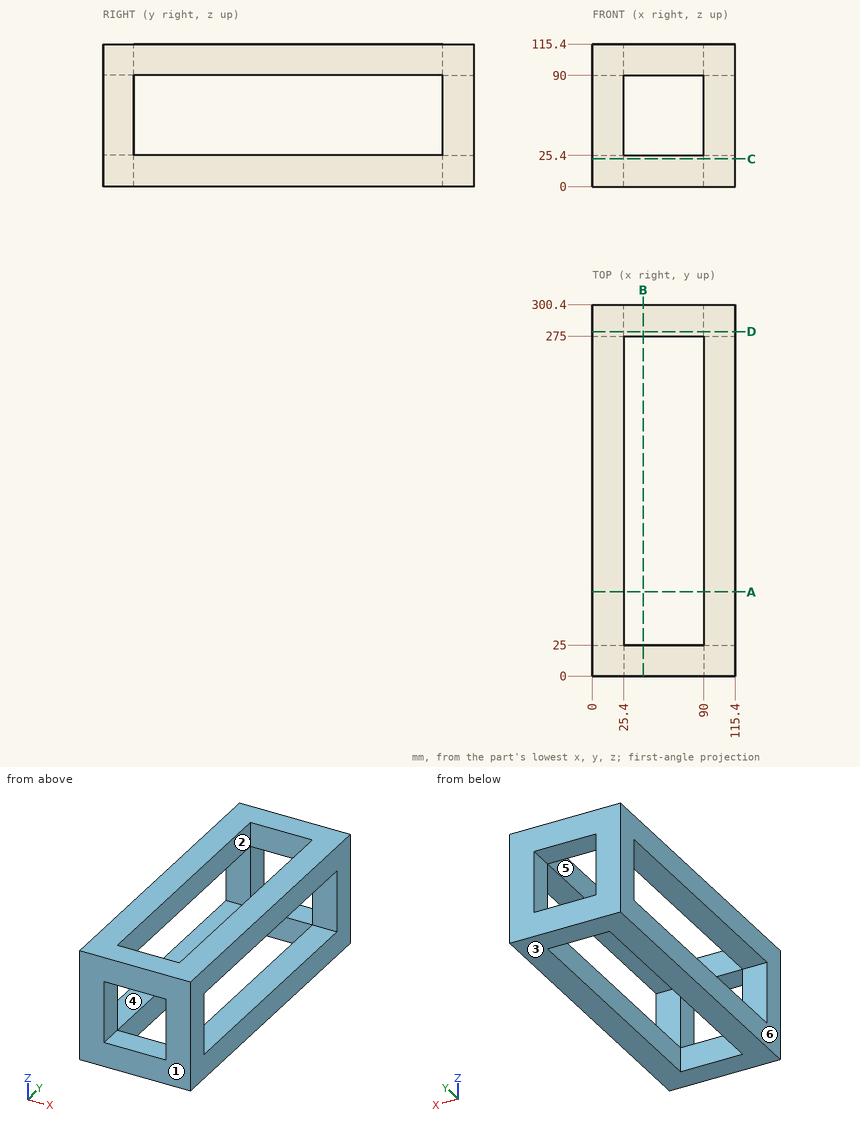
Input: dimensioned drawing with shaded views. Units: mm. Origin: part minimum x, y, z. A direction names the side the tool comes from. Coordinates: 2 decimals unless noted, no trailing zeros. Loops run counter-clockwise (first coordinate to the right, second up) from the corner with the lowest first, then second, coordinate; pieces in that order, holes last. Notation, with made-up numbers: (9, 44) -> (52, 44) arc R19 cw to (52, 53) -> close; hole circle Ø11 at (69.25, -5). An arc over 180 degrees is marked (long way). Use a Markdown table: item, result. Add a question column.
(1) Access query for the marked faces 4, 5 and 6. Directions: +Z, -Z, +X, -X, +Y, -Y. A direction counts if a zero-diameter tool reaches every point of the face in a straight line with its end or side. Return the directions, or none.
(2) Section query A-A, the plane y = 68. Return loops of the section in (x, z), plus the area to 3 significant figures.
(3) Section query D-D, the plane y = 278.5. Return loops of the section in (x, z).
(4) Section query B-B, the plane x = 41. Return loops of the section in (y, z), plus the area to 3 significant figures.
(5) Mould query, pull axis Y, two halves, no side actions, for the marked faces 1, 2 and 3. Classes: pulls with the +Y half, pulls with the -Y half, needs draft (parallel to the pull), parting line crosses it, or undercut.
(6) Line query: line 1 along Y through (x, z) = (78, 9); line 2 along X through (y, z) = (199, 110). Output: solid intervals per line, ascending.
(7) Section query C-C, the plane z = 22.5. Return loops of the section in (x, y).
Answer:
| question | item | result |
|---|---|---|
| 1 | face 4 | +X, -X |
| 1 | face 5 | +Z, -Z |
| 1 | face 6 | +Z, -Z, -X, +Y, -Y |
| 2 | outline | (0, 0) -> (25.4, 0) -> (25.4, 25.4) -> (0, 25.4) -> close; (0, 90) -> (25.4, 90) -> (25.4, 115.4) -> (0, 115.4) -> close; (90, 0) -> (115.4, 0) -> (115.4, 25.4) -> (90, 25.4) -> close; (90, 90) -> (115.4, 90) -> (115.4, 115.4) -> (90, 115.4) -> close |
| 2 | area | 2,580 mm^2 |
| 3 | outline | (0, 0) -> (115.4, 0) -> (115.4, 115.4) -> (0, 115.4) -> close; hole (25.4, 25.4) -> (90, 25.4) -> (90, 90) -> (25.4, 90) -> close |
| 4 | outline | (0, 0) -> (25, 0) -> (25, 25.4) -> (0, 25.4) -> close; (0, 90) -> (25, 90) -> (25, 115.4) -> (0, 115.4) -> close; (275, 0) -> (300.4, 0) -> (300.4, 25.4) -> (275, 25.4) -> close; (275, 90) -> (300.4, 90) -> (300.4, 115.4) -> (275, 115.4) -> close |
| 4 | area | 2,560 mm^2 |
| 5 | face 1 | pulls with the -Y half |
| 5 | face 2 | undercut |
| 5 | face 3 | needs draft |
| 6 | line 1 | y = 0 to 25, 275 to 300.4 |
| 6 | line 2 | x = 0 to 25.4, 90 to 115.4 |
| 7 | outline | (0, 0) -> (115.4, 0) -> (115.4, 300.4) -> (0, 300.4) -> close; hole (25.4, 25) -> (90, 25) -> (90, 275) -> (25.4, 275) -> close |
